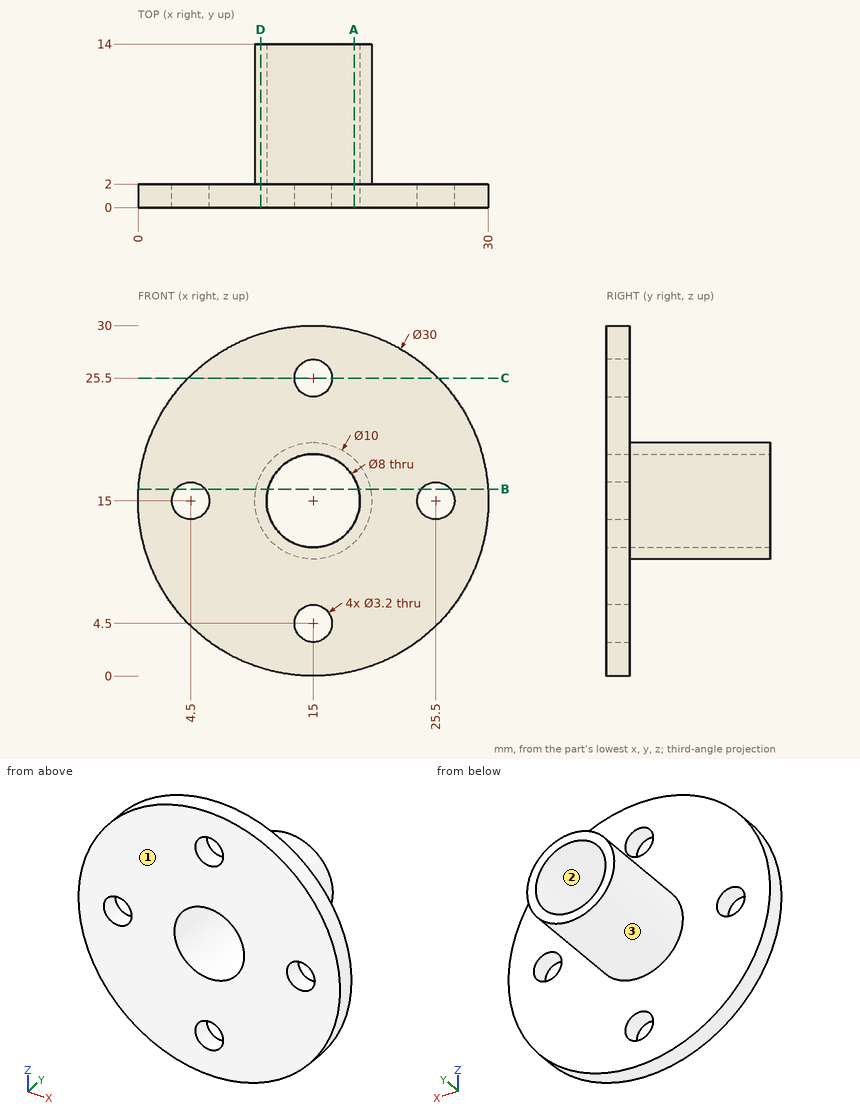
Study the drawing (mm; zero at the part's minimum x, y, z) and answer. Give positions to 0.01 mm unless a question says otherwise; leave off trailing zeros. Loops run counter-clockwise (first coordinate to the right, second up) from the corner with the lowest first, then second, coordinate; pieces in that order, holes last. Notation, with made-up numbers: (-15.5, 6.25) - (1.5, 6.25) arc R21 cw to (1.5, 12.25) - close; hole circle Ø11 at (17.5, 68). An arc over 180 degrees is marked (long way). Return JSON: item names as keys, results as strings. Group by question number.
1. Find section C-C (z = 25.5). Write down the section's boundary in (x, y), then the cut area to 3 significant figures.
2. Find section D-D (x = 10.5). Write down the section's boundary in (y, z).
3. Determine the mould class of the marked faces 1, 2 and 3 for opening direction X: pulls with the +X half, pulls with the -X half, needs draft (parallel to the pull), parting line crosses it, or undercut.
4. Find section B-B (z = 16). Write down the section's boundary in (x, y).
5. Find section A-A (x = 18.5). Write down the section's boundary in (y, z), then the cut area to 3 significant figures.
6. Given pin 1 Ø3 at (x, y) = (15, 7) entering from +Z; pin 2 Ø6 at (y, z) = (11.5, 11) entering from +X; pin 3 Ø1.5 at (x, z) = (13, 13) entering from +Y; pin 4 Ø2 at (x, y) = (9.5, 3.5) entering from -Z, each flat-ended and moving along its own axis, determine where each tip first touches the part or whether it passes through.
7. Straight lines are drawn through the part: line 1 (X direction, y = 1.5, z = 15); line 2 (X direction, y = 7.25, z = 15); line 3 (Y direction, x = 22, z = 25.75). For each, find the intervals that lie inside material, in ascending order. Write a range as [from, to].
Verdict:
{
 "1": {"outline": "(4.29, 0) - (13.4, 0) - (13.4, 2) - (4.29, 2) - close; (16.6, 0) - (25.71, 0) - (25.71, 2) - (16.6, 2) - close", "area": "36.4 mm^2"},
 "2": {"outline": "(0, 0.69) - (2, 0.69) - (2, 12.82) - (14, 12.82) - (14, 17.18) - (2, 17.18) - (2, 29.31) - (0, 29.31) - close"},
 "3": {"face 1": "needs draft", "face 2": "undercut", "face 3": "parting line crosses it"},
 "4": {"outline": "(0.03, 0) - (3.25, 0) - (3.25, 2) - (0.03, 2) - close; (5.75, 0) - (11.13, 0) - (11.13, 14) - (10.1, 14) - (10.1, 2) - (5.75, 2) - close; (18.87, 0) - (24.25, 0) - (24.25, 2) - (19.9, 2) - (19.9, 14) - (18.87, 14) - close; (26.75, 0) - (29.97, 0) - (29.97, 2) - (26.75, 2) - close"},
 "5": {"outline": "(0, 0.41) - (2, 0.41) - (2, 11.43) - (14, 11.43) - (14, 13.06) - (0, 13.06) - close; (0, 16.94) - (14, 16.94) - (14, 18.57) - (2, 18.57) - (2, 29.59) - (0, 29.59) - close", "area": "89.8 mm^2"},
 "6": {"pin 1": "stops at z = 20", "pin 2": "stops at x = 19.9", "pin 3": "passes through", "pin 4": "stops at z = 12.82"},
 "7": {"line 1": "x = [0, 2.9], [6.1, 11], [19, 23.9], [27.1, 30]", "line 2": "x = [10, 11], [19, 20]", "line 3": "y = [0, 2]"}
}
